The listing builds one solid part. Answer for the finished solid, in the listing's coordinates (mm). Face numbers are marked on the shaded views. A direction names the side the tool comes from. Round coordinates to 2 decimals unless told otherwise and drop trailing zeros. Loops run counter-clockwise (first coordinate to the right, second up) from the corner with the lowest first, then second, coordinate; pieces in that order, holes last. Notation, with made-up numbers: (-27.5, 36) -> (13.5, 36) arc R15 cw to (13.5, 64) -> close; hole circle Ø4 at (9, -37). An arc over 180 degrees is marked (long way). Answer in a Markdown table with one row per item. Add a question column.
```python
from build123d import *

# Parameters (mm, degrees)
F0_R     = 38.5018988787
F0_R_2   = 16.939934048
F1_DEPTH = 95
F5_W     = 37.283
F5_H     = 37.253003633
F6_DEPTH = 100
F7_R     = 13.5195959493


# Not quite as in the source:
# - a fillet or chamfer that OpenCascade refuses, or shapes differently, is made with other operations: its cross-section is extruded or revolved along the edge and cut away or added


with BuildPart() as f1:
    # F0 (on Top) → F1 (new body)
    with BuildSketch(Plane.XY):
        Circle(F0_R)
        Circle(F0_R_2, mode=Mode.SUBTRACT)
    extrude(amount=F1_DEPTH)

    # F5 (on line) → F6 (cut)
    with BuildSketch(Plane.YZ.offset(-38.5018988787)):
        with Locations((0, 37.3)):
            Rectangle(F5_W, F5_H)
    extrude(amount=F6_DEPTH, mode=Mode.SUBTRACT)

    # F7
    f7_edges = [f1.edges().sort_by_distance(p)[0] for p in [
        (-38.501899, 0, 95),
    ]]
    fillet(f7_edges, radius=F7_R)

    # F8: fillet of radius 29.8468724241 on 1 edges, made by hand

    # F8_s1 → F8_t2 (revolve, cut)
    with BuildSketch(Plane.XZ):
        with BuildLine():
            ThreePointArc((24.9823029294, 95), (19.0232329538, 85.5740041188), (16.939934048, 74.6186502225))
            Line((16.939934048, 74.6186502225), (16.939934048, 95))
            Line((16.939934048, 95), (24.9823029294, 95))
        make_face()
    revolve(axis=Axis((0, 0, 95), (0, 0, 1)), mode=Mode.SUBTRACT)


solid = f1.part
```
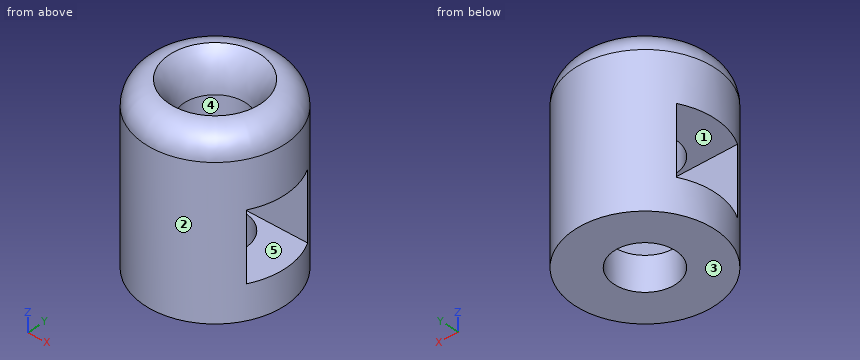
Item 1: For the marked faces 1 and 2, determine the directions among +Z, -Z, +X, -X, +Y, -Y from which every point of the face is accessible in a straight line to the end or side of a thin tool.
Item 2: The mould has two halves that part along Z. Classify the marked faces 3, 4 and 5: +Z half, -Z half, draft (parallel to the pull), parting line (faces both ways), or undercut.
Item 3: Consider L1, parallel to Y at x = 0, z = 4.25; L2, parallel to Y at x = 6.5, z = 49.5; L3, parallel to X at y = -4, z = 66. Determine where each line is inside the solid, lowest interval first. Write a range as from..to.
Item 4: Section C-C, the plane z = 51 is taken. Write down the section's boundary in (x, y), and give its area (3 significant figures).
Item 5: Flat-ended cylindrical pins translate along their axes: P1, Ø11, axis at x = -5.5, y = -9, coming from the +Z side; P2, Ø1.5, axis at x = 28.5, z = 59.5, coming from the +Y side; P3, Ø18.5, axis at x = -5.5, z = 33.5, coming from the +Y side; P4, Ø2, axis at y = -20, z = 39, coming from the +X side. Find the tip coordinate at first contact, or state that the pin passes through.
Item 6: Section A-A, the plane y = 0 is taken. Write down the section's boundary in (x, z).
Item 7: Section D-D, the plane z = 9.5 is taken. Write down the section's boundary in (x, y).
Item 8: Section B-B, the plane x = 0 is taken. Write down the section's boundary in (y, z).
Here are the results:
| question | item | result |
|---|---|---|
| 1 | face 1 | +X, -X |
| 1 | face 2 | +Z, -Z |
| 2 | face 3 | -Z half |
| 2 | face 4 | draft |
| 2 | face 5 | undercut |
| 3 | L1 | y = -38.5..-16.94, 16.94..38.5 |
| 3 | L2 | y = -37.95..-18.64, 18.64..37.95 |
| 3 | L3 | x = -38.29..-16.46, 16.46..38.29 |
| 4 | outline | (-33.69, -18.64) arc R38.5 ccw to (33.69, -18.64) -> close; (-33.69, 18.64) -> (33.69, 18.64) arc R38.5 ccw to start |
| 4 | area | 1,900 mm² |
| 5 | P1 | passes through |
| 5 | P2 | stops at y = 26.69 |
| 5 | P3 | stops at y = 38.5 |
| 5 | P4 | stops at x = 33.49 |
| 6 | outline | (-38.5, 0) -> (-16.94, 0) -> (-16.94, 18.67) -> (-38.5, 18.67) -> close; (-38.5, 55.93) -> (-16.94, 55.93) -> (-16.94, 74.62) arc R29.85 ccw to (-24.98, 95) arc R13.52 ccw to (-38.5, 81.48) -> close; (16.94, 0) -> (38.5, 0) -> (38.5, 18.67) -> (16.94, 18.67) -> close; (16.94, 55.93) -> (38.5, 55.93) -> (38.5, 81.48) arc R13.52 ccw to (24.98, 95) arc R29.85 ccw to (16.94, 74.62) -> close |
| 7 | outline | circle Ø77 at (0, 0); hole circle Ø33.88 at (0, 0) |
| 8 | outline | (-38.5, 0) -> (-16.94, 0) -> (-16.94, 18.67) -> (-18.64, 18.67) -> (-18.64, 55.93) -> (-16.94, 55.93) -> (-16.94, 74.62) arc R29.85 ccw to (-24.98, 95) arc R13.52 ccw to (-38.5, 81.48) -> close; (16.94, 0) -> (38.5, 0) -> (38.5, 81.48) arc R13.52 ccw to (24.98, 95) arc R29.85 ccw to (16.94, 74.62) -> (16.94, 55.93) -> (18.64, 55.93) -> (18.64, 18.67) -> (16.94, 18.67) -> close |
